Read the model definition and answer for the solid it produces. Units are mm, in the model's axes. Face numbers are marked on the shaded views. A direction names the side the tool comes from. Give positions to 0.01 mm unless a question says otherwise; leave off trailing zeros. Loops run counter-clockwise (first coordinate to the right, second up) from the corner with the lowest first, then second, coordinate; pieces in that order, holes last. Notation, with made-up numbers: (-28, 71.5) -> (4, 71.5) arc R13 cw to (4, 95.5) -> close; hole circle Ø11 at (22, -30.75). An arc over 180 degrees is marked (long way). Write each question's results on one line, items separated by ' | '. Start each with the question number.
Item 1: Section B-B on x = -14.5 is taken. Write down the section's boundary in (y, z), and give its area (3 significant figures).
Item 2: Section A-A on z = 11.5 is taken. Write down the section's boundary in (x, y), and give its area (3 significant figures).
Item 3: Find the intervals of material crossed by line 1 (X direction, y = -13, z = 11.75); line 2 (Y direction, x = 16, z = 10.5); line 3 (Z direction, x = -26.5, y = -14), in increasing order.
Item 4: Section C-C on y = 10 is taken. Write down the section's boundary in (x, z), and give its area (3 significant figures).
Item 5: Determine the mould class of the marked faces 1, 2 and 3 for opening direction Y: +Y half, -Y half, draft (parallel to the pull), parting line (faces both ways), or undercut.
Item 6: This flat-tipped pin is pushed along its axis until it touches: P1, Ø3, axis at x = -8.5, y = -6.5, coming from the +Z side. Where does it stop, or does it pass through?
Item 7: Which of the six approach directions +Z, -Z, +X, -X, +Y, -Y give full straight-line access (tool end or side, diameter ignored) to the marked faces 4 and 5?
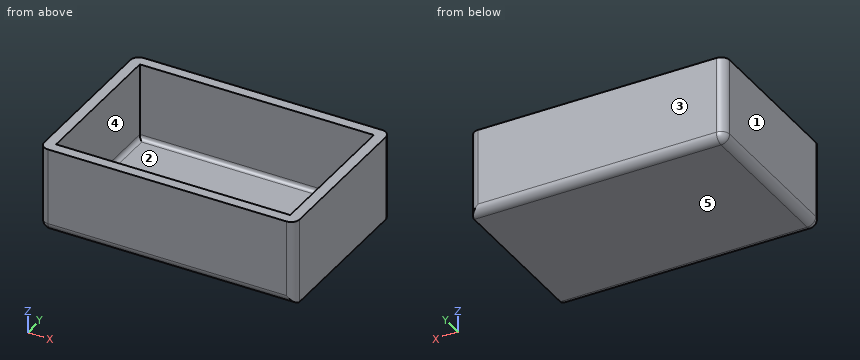
```python
from build123d import *

# Parameters (mm, degrees)
SKETCH1_W           = 60
SKETCH1_H           = 40
BOSS_EXTRUDE1_DEPTH = 20
SKETCH2_W           = 55
SKETCH2_H           = 35
CUT_EXTRUDE1_DEPTH  = 18
FILLET1_R           = 1
FILLET2_R           = 2


with BuildPart() as part:
    # Sketch1 → Boss-Extrude1 (new body)
    with BuildSketch(Plane.XY):
        Rectangle(SKETCH1_W, SKETCH1_H)
    extrude(amount=BOSS_EXTRUDE1_DEPTH)

    # Sketch2 → Cut-Extrude1 (cut)
    with BuildSketch(Plane.XY.offset(20)):
        Rectangle(SKETCH2_W, SKETCH2_H)
    extrude(amount=-CUT_EXTRUDE1_DEPTH, mode=Mode.SUBTRACT)

    # Fillet1
    fillet1_edges = [part.edges().sort_by_distance(p)[0] for p in [
        (27.5, 0, 2),
        (0, -17.5, 2),
        (-27.5, 0, 2),
        (0, 17.5, 2),
    ]]
    fillet(fillet1_edges, radius=FILLET1_R)

    # Fillet2
    fillet2_edges = [part.edges().sort_by_distance(p)[0] for p in [
        (0, -20, 0),
        (-30, 0, 0),
        (0, 20, 0),
        (30, -20, 10),
        (-30, -20, 10),
        (-30, 20, 10),
        (30, 20, 10),
    ]]
    fillet(fillet2_edges, radius=FILLET2_R)


solid = part.part
```
Findings:
1) outline: (-20, 2) arc R2 ccw to (-18, 0) -> (18, 0) arc R2 ccw to (20, 2) -> (20, 20) -> (17.5, 20) -> (17.5, 3) arc R1 cw to (16.5, 2) -> (-16.5, 2) arc R1 cw to (-17.5, 3) -> (-17.5, 20) -> (-20, 20) -> close | area: 169 mm2
2) outline: (-30, -18) arc R2 ccw to (-28, -20) -> (28, -20) arc R2 ccw to (30, -18) -> (30, 18) arc R2 ccw to (28, 20) -> (-28, 20) arc R2 ccw to (-30, 18) -> close; hole (-27.5, -17.5) -> (27.5, -17.5) -> (27.5, 17.5) -> (-27.5, 17.5) -> close | area: 472 mm2
3) line 1: -30 to -27.5, 27.5 to 30 | line 2: -20 to -17.5, 17.5 to 20 | line 3: 0 to 2
4) outline: (-30, 2) arc R2 ccw to (-28, 0) -> (30, 0) -> (30, 20) -> (27.5, 20) -> (27.5, 3) arc R1 cw to (26.5, 2) -> (-26.5, 2) arc R1 cw to (-27.5, 3) -> (-27.5, 20) -> (-30, 20) -> close | area: 210 mm2
5) face 1: draft | face 2: undercut | face 3: +Y half
6) P1: z = 2
7) face 4: +Z | face 5: -Z, +X, -X, +Y, -Y
